Geometry: see drawing. Coordinates: mm, zero at the bounding-box minimum. A direction names the side the tool comes from. Round coordinates to 2 decimals unless told otherwise and drop trailing zeros. Write each loop counter-clockwise with the first axis right and the second up, starting at its lowest first coordinate (ties: lowest second). Pieces come first, ordered by that corner, then holes. Notation, with made-up numbers: M -27.5,5 L 23.5,5 A26 cw 23.5,25 Z; hole C 55,73 d6. An arc over 180 degrees is marked long. Use one line per item in the form item = value. Start each with the question number.
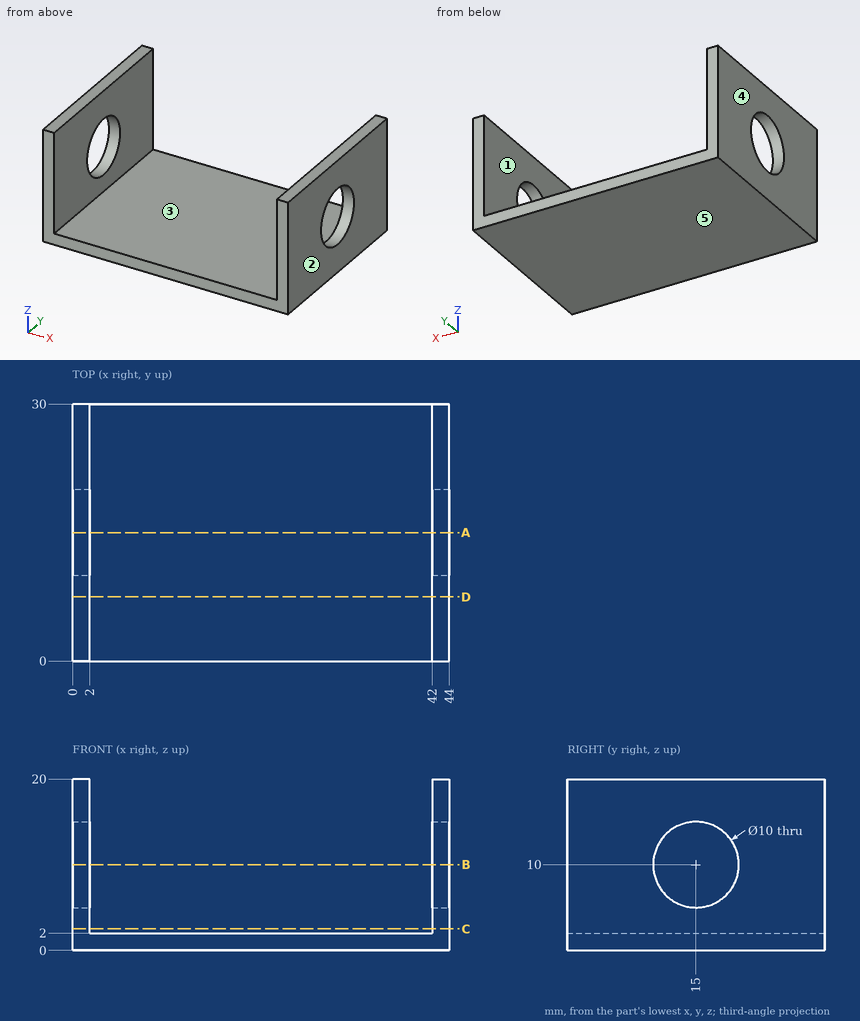
Item 1: Cut plane A-A (y = 15). Output: boundary loops of the cut face in (x, z).
Item 2: Cut plane C-C (z = 2.5). Output: boundary loops of the cut face in (x, y), plus the area to 3 significant figures.
Item 3: Cut plane B-B (z = 10). Output: boundary loops of the cut face in (x, y), plus the area to 3 significant figures.
Item 4: Reachability of the marked faces 1 and 2 from +Z, -Z, +X, -X, +Y, -Y: full face, straight path, thin tool, end or side. Return the list, or none.
Item 5: Ray query, line 1 (Z direction, x = 42.7, y = 15); line 2 (X direction, y = 4, z = 5.25); line 3 (Z direction, x = 11, y = 17). Return the intervals inside material, ascending. Write a range as from..to.
Item 6: First-contact query: pin 1 (6 mm diameter, centred on x = 21, y = 10, fed in from +Z); pin 2 (8 mm diameter, centred on y = 15, z = 10, fed in from +X) (3 decimals). Flat tips, straight axial feed; report the tip coordinate or a pass-through.
Item 7: Cut plane D-D (y = 7.5). Output: boundary loops of the cut face in (x, z).
Item 8: Draft query along X for the marked faces 3, 4 and 5. Return one class per face: +X half, -X half, draft (parallel to the pull), parting line (faces both ways), or undercut.
Final values:
q1.outline = M 0,0 L 44,0 L 44,5 L 42,5 L 42,2 L 2,2 L 2,5 L 0,5 Z; M 0,15 L 2,15 L 2,20 L 0,20 Z; M 42,15 L 44,15 L 44,20 L 42,20 Z
q2.outline = M 0,0 L 2,0 L 2,30 L 0,30 Z; M 42,0 L 44,0 L 44,30 L 42,30 Z
q2.area = 120 mm^2
q3.outline = M 0,0 L 2,0 L 2,10 L 0,10 Z; M 0,20 L 2,20 L 2,30 L 0,30 Z; M 42,0 L 44,0 L 44,10 L 42,10 Z; M 42,20 L 44,20 L 44,30 L 42,30 Z
q3.area = 80.0 mm^2
q4.face_1 = +Z, +Y, -Y
q4.face_2 = +Z, -Z, +X, +Y, -Y
q5.line_1 = 0..5, 15..20
q5.line_2 = 0..2, 42..44
q5.line_3 = 0..2
q6.pin_1 = 2
q6.pin_2 = through
q7.outline = M 0,0 L 44,0 L 44,20 L 42,20 L 42,2 L 2,2 L 2,20 L 0,20 Z
q8.face_3 = undercut
q8.face_4 = -X half
q8.face_5 = draft
